```python
from build123d import *

# Parameters (mm, degrees)
SKETCH1_R           = 65
SKETCH1_R_2         = 17.5
BOSS_EXTRUDE2_DEPTH = 1
BOSS_EXTRUDE3_START = 3
SKETCH2_R           = 65
BOSS_EXTRUDE3_DEPTH = 3
SKETCH3_R           = 5
CUT_EXTRUDE1_DEPTH  = 128.342059038
SKETCH4_R           = 2.5
CUT_EXTRUDE2_DEPTH  = 128.342059038


with BuildPart() as part:
    # Sketch1 → Boss-Extrude2 (new body)
    with BuildSketch(Plane(origin=(0, 0, 0), x_dir=(1, 0, 0), z_dir=(0, 1, 0))):
        with Locations(Location((25, -25, 0), (0, 0, 270))):
            Circle(SKETCH1_R)
        with Locations(Location((0, 0, 0), (0, 0, 270))):
            Circle(SKETCH1_R_2, mode=Mode.SUBTRACT)
        with Locations(Location((50, 0, 0), (0, 0, 270))):
            Circle(SKETCH1_R_2, mode=Mode.SUBTRACT)
        with Locations(Location((50, -50, 0), (0, 0, 270))):
            Circle(SKETCH1_R_2, mode=Mode.SUBTRACT)
        with Locations(Location((0, -50, 0), (0, 0, 270))):
            Circle(SKETCH1_R_2, mode=Mode.SUBTRACT)
    extrude(amount=BOSS_EXTRUDE2_DEPTH)

    # Sketch2 → Boss-Extrude3 (add)
    with BuildSketch(Plane.XZ.offset(BOSS_EXTRUDE3_START)):
        with Locations(Location((25, 25, 0), (0, 0, 270))):
            Circle(SKETCH2_R)
    extrude(amount=-BOSS_EXTRUDE3_DEPTH)

    # Sketch3 → Cut-Extrude1 (cut, through all)
    with BuildSketch(Plane(origin=(0, 1, 0), x_dir=(1, 0, 0), z_dir=(0, 1, 0))):
        with Locations(Location((25, 15, 0), (0, 0, 270))):
            Circle(SKETCH3_R)
        with Locations(Location((65, -25, 0), (0, 0, 270))):
            Circle(SKETCH3_R)
        with Locations(Location((25, -65, 0), (0, 0, 270))):
            Circle(SKETCH3_R)
        with Locations(Location((-15, -25, 0), (0, 0, 270))):
            Circle(SKETCH3_R)
    extrude(amount=-CUT_EXTRUDE1_DEPTH, mode=Mode.SUBTRACT)

    # Sketch4 → Cut-Extrude2 (cut, through all)
    with BuildSketch(Plane(origin=(0, 1, 0), x_dir=(1, 0, 0), z_dir=(0, 1, 0))):
        with Locations(Location((25, 32.5, 0), (0, 0, 270))):
            Circle(SKETCH4_R)
        with Locations(Location((82.5, -25, 0), (0, 0, 270))):
            Circle(SKETCH4_R)
        with Locations(Location((25, -82.5, 0), (0, 0, 270))):
            Circle(SKETCH4_R)
        with Locations(Location((-32.5, -25, 0), (0, 0, 270))):
            Circle(SKETCH4_R)
    extrude(amount=-CUT_EXTRUDE2_DEPTH, mode=Mode.SUBTRACT)


solid = part.part
```
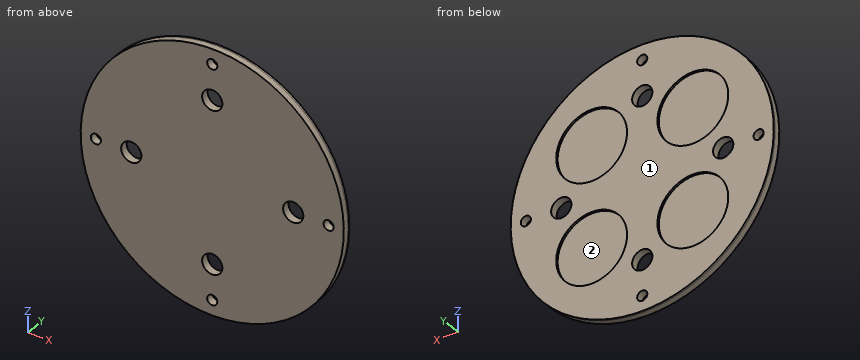
Build history of the part. All positions in model axes, mm. Face numbers are marked on the shaded views. A direction names the side the tool comes from. Give positions to 0.01 mm unless a question says otherwise; leave off trailing zeros. Loops run counter-clockwise (first coordinate to the right, second up) from the corner with the lowest first, then second, coordinate; pieces in that order, holes last.
Item 1: Flat gauge pins, fed straight in: pin 1 (1 mm diameter, centred on x = 19, y = -1, fed in from +Z); pin 2 (13 mm diameter, centred on x = 25, z = 65, fed in from +Y); pin 3 (10.5 mm diameter, centred on x = -4, z = 44, fed in from +Y). Where does each tip first touch, or does it go through?
Answers follow:
pin 1: stops at z = 89.77
pin 2: stops at y = 1
pin 3: stops at y = 0
Item 2: Slice it at D-D, the plane z = 63. List the corners of the cut face in (x, y).
Answers follow:
outline: (-27.74, -3) - (20.42, -3) - (20.42, 1) - (11.72, 1) - (11.72, 0) - (-11.72, 0) - (-11.72, 1) - (-27.74, 1) - close; (29.58, -3) - (77.74, -3) - (77.74, 1) - (61.72, 1) - (61.72, 0) - (38.28, 0) - (38.28, 1) - (29.58, 1) - close
Item 3: Drill centre lines: line 1 (X direction, y = -1.65, z = 25); line 2 (X direction, y = 0.6, z = 50); line 3 (Z direction, x = 62.5, y = 0.5). Where is each one in solid material? Low to high.
Answers follow:
line 1: x = -40 to -35, -30 to -20, -10 to 60, 70 to 80, 85 to 90
line 2: x = -35 to -17.5, 17.5 to 32.5, 67.5 to 85
line 3: z = -28.09 to -12.25, 12.25 to 20.67, 29.33 to 37.75, 62.25 to 78.09
Item 4: Slice it at B-B, the plane y = -1.6. Give the number of separate pieces and of enclosed holes in the cut face, and give its area (3 significant figures).
Answers follow:
separate pieces: 1
enclosed holes: 8
area: 12,900 mm2
Item 5: Which spindle directions (+Z, -Z, +X, -X, +Y, -Y) get a long thin tool onto all of the face, cutting with end or side? Do the marked faces 1 and 2. Say none if no direction does.
Answers follow:
face 1: +Z, -Z, +X, -X, +Y
face 2: +Y
Item 6: Slice it at A-A, the plane z = 25. List the corners of the cut face in (x, y).
Answers follow:
outline: (-40, -3) - (-35, -3) - (-35, 1) - (-40, 1) - close; (-30, -3) - (-20, -3) - (-20, 1) - (-30, 1) - close; (-10, -3) - (60, -3) - (60, 1) - (-10, 1) - close; (70, -3) - (80, -3) - (80, 1) - (70, 1) - close; (85, -3) - (90, -3) - (90, 1) - (85, 1) - close
Item 7: Slice it at C-C, the plane x = -32.5. List the corners of the cut face in (y, z), and give its area (3 significant figures).
Answers follow:
outline: (-3, -5.31) - (1, -5.31) - (1, 22.5) - (-3, 22.5) - close; (-3, 27.5) - (1, 27.5) - (1, 55.31) - (-3, 55.31) - close
area: 222 mm2
